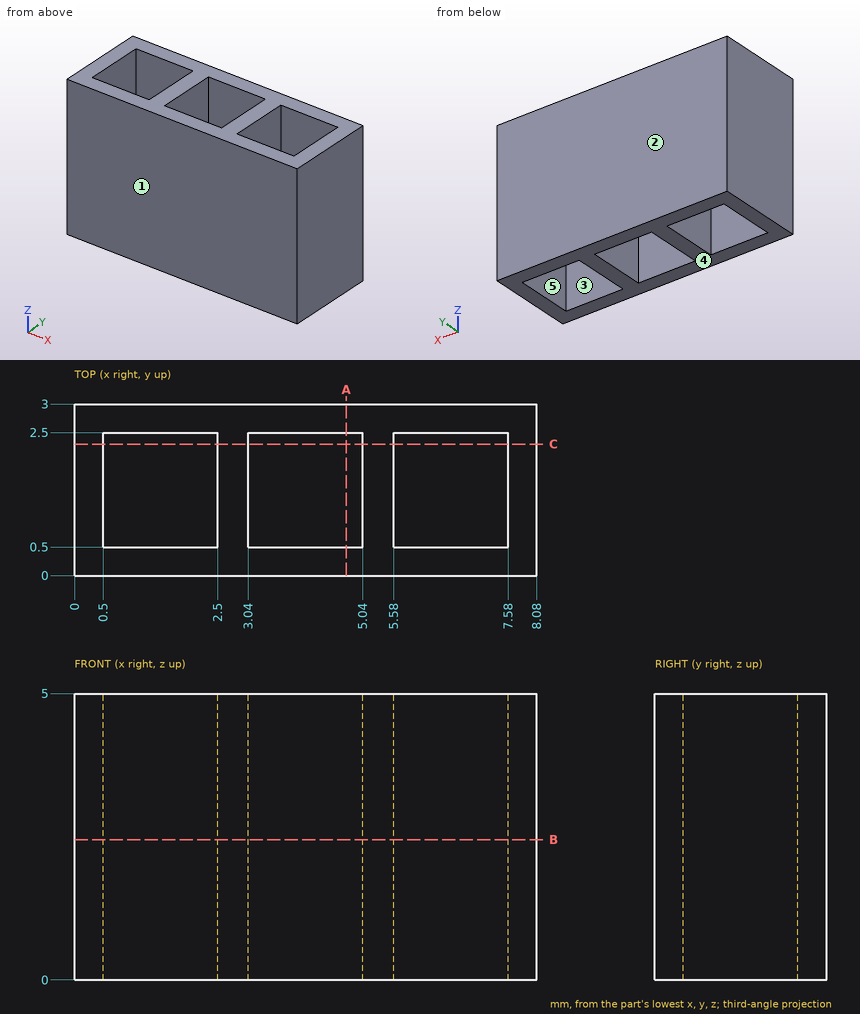
Answer from the drawing. Dimensions are ordinates in mm from the lowest x, y and z of the part. A direction names the side the tool comes from. Coordinates: 2 decimals unless noted, no trailing zeros. Write each loop counter-clockwise with the first axis right and the second up, starting at its lowest first coordinate (ties: lowest second). Pieces come first, ordered by that corner, then holes. Notation, with made-up numbers: M -4.75,83.25 L 39.25,83.25 A19 ccw 39.25,117.25 Z; hole C -36,39.25 d3. An arc over 180 degrees is marked long. Use a Markdown table: item, result.
Q1. This flat-tipped pin is pushed along its axis until it touches: pin 1 Ø1 at (x, y) = (4, 1.5) entering from -Z. Where does it stop, or does it pass through?
Answer block:
| item | result |
|---|---|
| pin 1 | passes through |
Q2. The part is cut by section B-B, the plane z = 2.45. Write down the section's boundary in (x, y).
Answer block:
| item | result |
|---|---|
| outline | M 0,0 L 8.08,0 L 8.08,3 L 0,3 Z; hole M 0.5,0.5 L 2.5,0.5 L 2.5,2.5 L 0.5,2.5 Z; hole M 3.04,0.5 L 5.04,0.5 L 5.04,2.5 L 3.04,2.5 Z; hole M 5.58,0.5 L 7.58,0.5 L 7.58,2.5 L 5.58,2.5 Z |
Q3. Determine the mould class of the marked faces 1, 2 and 3 for opening direction Y: released by +Y, released by -Y, zero draft, split by the parting line, or undercut.
Answer block:
| item | result |
|---|---|
| face 1 | released by -Y |
| face 2 | released by +Y |
| face 3 | undercut |
Q4. Straight lines are drawn through the part: L1, parallel to X at y = 0.7, z = 4; L2, parallel to Y at x = 1.75, z = 2.4. For each, find the intervals that lie inside material, in ascending order. Write a range as [from, to].
Answer block:
| item | result |
|---|---|
| L1 | x = [0, 0.5], [2.5, 3.04], [5.04, 5.58], [7.58, 8.08] |
| L2 | y = [0, 0.5], [2.5, 3] |
Q5. The part is cut by section C-C, the plane y = 2.3. Write down the section's boundary in (x, z).
Answer block:
| item | result |
|---|---|
| outline | M 0,0 L 0.5,0 L 0.5,5 L 0,5 Z; M 2.5,0 L 3.04,0 L 3.04,5 L 2.5,5 Z; M 5.04,0 L 5.58,0 L 5.58,5 L 5.04,5 Z; M 7.58,0 L 8.08,0 L 8.08,5 L 7.58,5 Z |
Q6. Which of the six approach directions +Z, -Z, +X, -X, +Y, -Y give full straight-line access (tool end or side, diameter ignored) to the marked faces 4 and 5?
Answer block:
| item | result |
|---|---|
| face 4 | -Z, +X, -X, +Y, -Y |
| face 5 | +Z, -Z |
Q7. The part is cut by section A-A, the plane x = 4.75. Write down the section's boundary in (y, z).
Answer block:
| item | result |
|---|---|
| outline | M 0,0 L 0.5,0 L 0.5,5 L 0,5 Z; M 2.5,0 L 3,0 L 3,5 L 2.5,5 Z |
